Read the model definition and answer for the solid it produces. Units are mm, in the model's axes. Face numbers are marked on the shaded views. A direction names the side the tool comes from. Coordinates: 2 decimals unless noted, no trailing zeros. Write each loop counter-clockwise with the first axis right and the second up, starting at its lowest first coordinate (ties: lowest second). Pieces come first, ordered by that corner, then holes. Notation, with made-up numbers: (-19, 21) -> (27, 21) arc R31 cw to (27, 48) -> close; hole circle Ø11 at (18, 16). An arc over 180 degrees is marked (long way). Answer as a JSON object with one key per item and string values. Group by question number.
(1) A flat-ended cylindrical pin translates along its axis: P1, Ø8, axis at x = 1, y = -0.5, coming from the +Z side. Find the tip coordinate at first contact, or state that the pin passes through.
(2) Find section D-D (x = 0). Give the vertices of the cut face in (y, z), then the cut area to 4 significant figures.
(3) Find section A-A (x = 20). Give the vertices of the cut face in (y, z).
(4) For a pull along Y with two mould halves and no side action, classify the marked faces 3, 4 and 5 as +Y half, -Y half, draft (parallel to the pull), parting line (faces both ways), or undercut.
(5) Find section B-B (z = 3). Give the vertices of the cut face in (x, y).
(6) Straight lines are drawn through the part: L1, parallel to Y at x = 20, z = 4; L2, parallel to Y at x = 0, z = 7.45; L3, parallel to X at y = 4, z = 3.5. For each, find the intervals that lie inside material, in ascending order.
(7) Which of the six approach directions +Z, -Z, +X, -X, +Y, -Y give full straight-line access (tool end or side, diameter ignored) to the marked faces 1 and 2?
(8) Find section C-C (y = 6.5). Give the vertices of the cut face in (x, z), then the cut area to 3 significant figures.
from build123d import *

# Parameters (mm, degrees)
SKETCH1_W           = 50
SKETCH1_H           = 20
BOSS_EXTRUDE1_DEPTH = 10
SKETCH3_R           = 8.05
CUT_EXTRUDE1_DEPTH  = 5
SKETCH5_R           = 2
CUT_EXTRUDE2_DEPTH  = 10


with BuildPart() as part:
    # Sketch1 → Boss-Extrude1 (new body)
    with BuildSketch(Plane.XY):
        Rectangle(SKETCH1_W, SKETCH1_H)
    extrude(amount=BOSS_EXTRUDE1_DEPTH)

    # Sketch3 → Cut-Extrude1 (cut)
    with BuildSketch(Plane.XY.offset(10)):
        Circle(SKETCH3_R)
    extrude(amount=-CUT_EXTRUDE1_DEPTH, mode=Mode.SUBTRACT)

    # Sketch5 → Cut-Extrude2 (cut)
    with BuildSketch(Plane(origin=(0, 0, 0), x_dir=(-1, 0, 0), z_dir=(0, 0, -1))):
        with Locations((-20, 5)):
            Circle(SKETCH5_R)
        with Locations((-20, -5)):
            Circle(SKETCH5_R)
        with Locations((20, 5)):
            Circle(SKETCH5_R)
        with Locations((20, -5)):
            Circle(SKETCH5_R)
    extrude(amount=-CUT_EXTRUDE2_DEPTH, mode=Mode.SUBTRACT)


solid = part.part
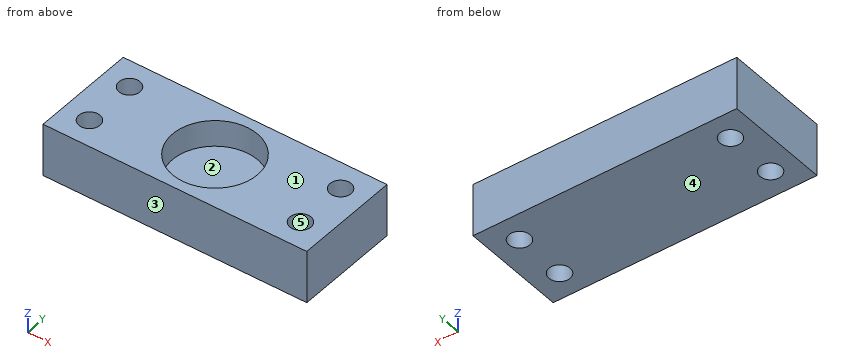
Results below:
{
 "1": {"P1": "stops at z = 5"},
 "2": {"outline": "(-10, 0) -> (10, 0) -> (10, 10) -> (8.05, 10) -> (8.05, 5) -> (-8.05, 5) -> (-8.05, 10) -> (-10, 10) -> close", "area": "119.5 mm2"},
 "3": {"outline": "(-10, 0) -> (-7, 0) -> (-7, 10) -> (-10, 10) -> close; (-3, 0) -> (3, 0) -> (3, 10) -> (-3, 10) -> close; (7, 0) -> (10, 0) -> (10, 10) -> (7, 10) -> close"},
 "4": {"face 3": "-Y half", "face 4": "draft", "face 5": "undercut"},
 "5": {"outline": "(-25, -10) -> (25, -10) -> (25, 10) -> (-25, 10) -> close; hole circle Ø4 at (-20, -5); hole circle Ø4 at (-20, 5); hole circle Ø4 at (20, -5); hole circle Ø4 at (20, 5)"},
 "6": {"L1": "y = -10 to -7, -3 to 3, 7 to 10", "L2": "y = -10 to -8.05, 8.05 to 10", "L3": "x = -25 to -21.73, -18.27 to 18.27, 21.73 to 25"},
 "7": {"face 1": "+Z, +X, -X, +Y, -Y", "face 2": "+Z"},
 "8": {"outline": "(-25, 0) -> (-21.32, 0) -> (-21.32, 10) -> (-25, 10) -> close; (-18.68, 0) -> (18.68, 0) -> (18.68, 10) -> (4.75, 10) -> (4.75, 5) -> (-4.75, 5) -> (-4.75, 10) -> (-18.68, 10) -> close; (21.32, 0) -> (25, 0) -> (25, 10) -> (21.32, 10) -> close", "area": "400 mm2"}
}
